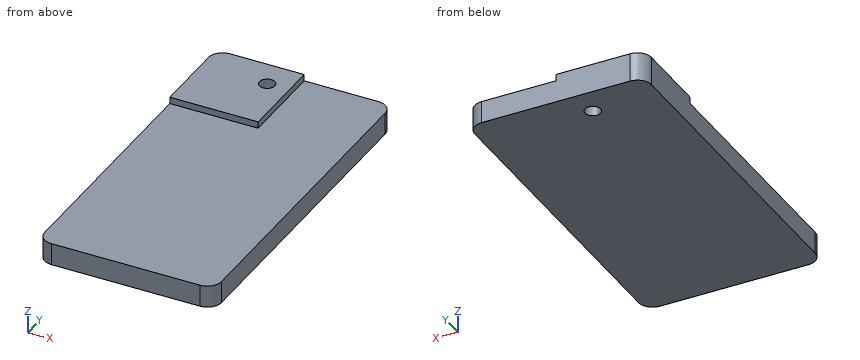
from build123d import *

# Parameters (mm, degrees)
SKETCH1_W           = 80
SKETCH1_H           = 155
BOSS_EXTRUDE1_DEPTH = 5
SKETCH2_W           = 40
SKETCH2_H           = 40
BOSS_EXTRUDE2_DEPTH = 3
SKETCH3_R           = 3.5
CUT_EXTRUDE1_DEPTH  = 89.177378051
FILLET1_R           = 6.35


with BuildPart() as part:
    # Sketch1 → Boss-Extrude1 (new, symmetric)
    with BuildSketch(Plane.XY):
        Rectangle(SKETCH1_W, SKETCH1_H)
    extrude(amount=BOSS_EXTRUDE1_DEPTH, both=True)

    # Sketch2 → Boss-Extrude2 (add)
    with BuildSketch(Plane.XY.offset(5)):
        with Locations((-20, 57.5)):
            Rectangle(SKETCH2_W, SKETCH2_H)
    extrude(amount=BOSS_EXTRUDE2_DEPTH)

    # Sketch3 → Cut-Extrude1 (cut, through all)
    with BuildSketch(Plane.XY.offset(8)):
        with Locations((-10, 64.5)):
            Circle(SKETCH3_R)
    extrude(amount=-CUT_EXTRUDE1_DEPTH, mode=Mode.SUBTRACT)

    # Fillet1
    fillet1_edges = [part.edges().sort_by_distance(p)[0] for p in [
        (40, -77.5, 0),
        (-40, -77.5, 0),
        (-40, 77.5, 1.5),
        (40, 77.5, 0),
    ]]
    fillet(fillet1_edges, radius=FILLET1_R)


solid = part.part
Design review of the part built by this model. Coordinates are the model's own, in mm. Coordinates: 2 decimals unless noted, no trailing zeros. Order: outer loops, then holes, each group sorted by start corner. A loop starts at its lowest first (then second) coordinate and runs counter-clockwise, first axis right, second up. Notation, with made-up numbers: (-23.75, 57.5) -> (-5.75, 57.5) arc R23 cw to (-5.75, 73.5) -> close; hole circle Ø10 at (88, -24). An arc over 180 degrees is marked (long way). Use one line per item in the form item = value. Start each with the question number.
(1) Insertion check: pin 1 (10 mm diameter, centred on x = 0.5, y = -25, fed in from +Z); pin 2 (0.9 mm diameter, centred on x = -11.5, z = 7, fed in from -Y); pin 3 (2.5 mm diameter, centred on y = 51.5, z = 7, fed in from +X). Each pin has a flat end and moves straight along its axis. Give the tip position at first contact, or say it passes through.
(2) Add section A-A on y = 64.5. State the section outline as (x, z) points.
(3) Add section C-C on x = 29. State the section outline as (y, z) points, plus the area to 3 significant figures.
(4) Add section B-B on x = -10. State the section outline as (y, z) points.
(5) For probe 1 along Y at (x, z) = (-10, 1.5); probe 2 along Y at (x, z) = (-10, 5.75); probe 3 along Z at (x, y) = (29.5, -40), list the stretches that pass through material, from the lowest coordinate up.
(6) Add section D-D on y = -43.5. State the section outline as (x, z) points.
Answer block:
q1.pin_1 = 5
q1.pin_2 = 37.5
q1.pin_3 = 0
q2.outline = (-40, -5) -> (-13.5, -5) -> (-13.5, 8) -> (-40, 8) -> close; (-6.5, -5) -> (40, -5) -> (40, 5) -> (0, 5) -> (0, 8) -> (-6.5, 8) -> close
q3.outline = (-77.5, -5) -> (77.5, -5) -> (77.5, 5) -> (-77.5, 5) -> close
q3.area = 1,550 mm²
q4.outline = (-77.5, -5) -> (61, -5) -> (61, 8) -> (37.5, 8) -> (37.5, 5) -> (-77.5, 5) -> close; (68, -5) -> (77.5, -5) -> (77.5, 8) -> (68, 8) -> close
q5.probe_1 = -77.5 to 61, 68 to 77.5
q5.probe_2 = 37.5 to 61, 68 to 77.5
q5.probe_3 = -5 to 5
q6.outline = (-40, -5) -> (40, -5) -> (40, 5) -> (-40, 5) -> close
